The drawing under review shows one solid part. Ordinate dimensions are in mm from its lowest x, y, z. Coordinates: 2 decimals unless noted, no trailing zeros. Write each loop counter-clockwise with the first axis right and the second up, starting at its lowest first coordinate (ties: lowest second). Pieces come first, ordered by that corner, then holes. Notation, with made-up numbers: (67, 1.25) - (87, 1.25) arc R20 ccw to (87, 8.25) - close; hole circle Ø11 at (-17.75, -18). An arc over 180 degrees is marked (long way). Use a Markdown table: item, result.
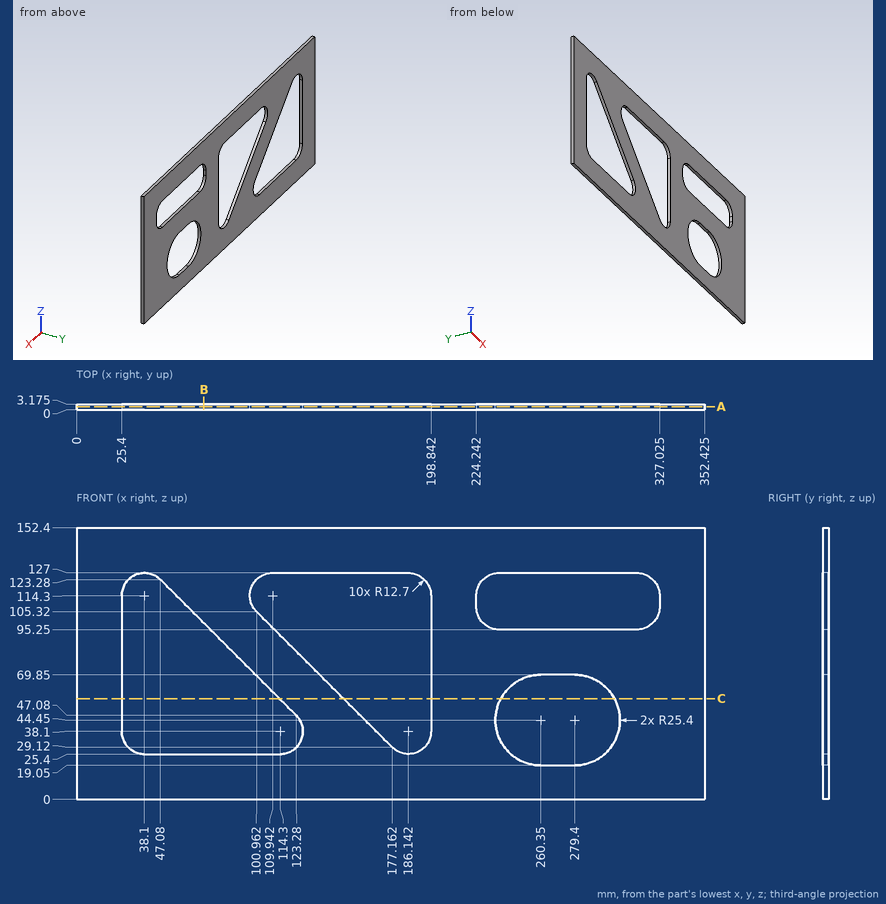
(1) Take a section at B-B on x = 71.5. Write out the cut boundary in (y, z) (1 decimal).
Determined:
| item | result |
|---|---|
| outline | (0, 0) - (3.2, 0) - (3.2, 25.4) - (0, 25.4) - close; (0, 98.9) - (3.2, 98.9) - (3.2, 152.4) - (0, 152.4) - close |
(2) For L1, parallel to X at y = 0.2, z = 97.5 (1 decimal); L2, parallel to X at y = 0.6, z = 29 (1 decimal); L3, parallel to X at y = 0.55, z = 73.5 (1 decimal), list the stretches that pass through material, from the lowest coordinate up. Write a range as from..to.
Determined:
| item | result |
|---|---|
| L1 | 0..25.4, 72.9..108.8, 198.8..229.7, 321.5..352.4 |
| L2 | 0..29.2, 123.2..177.3, 195..240.2, 299.6..352.4 |
| L3 | 0..25.4, 96.9..132.8, 198.8..352.4 |
(3) Take a section at C-C on z = 56.5. Write out the cut boundary in (x, y) (1 decimal), and give its area (3 significant figures).
Determined:
| item | result |
|---|---|
| outline | (0, 0) - (25.4, 0) - (25.4, 3.2) - (0, 3.2) - close; (113.9, 0) - (149.8, 0) - (149.8, 3.2) - (113.9, 3.2) - close; (198.8, 0) - (238, 0) - (238, 3.2) - (198.8, 3.2) - close; (301.8, 0) - (352.4, 0) - (352.4, 3.2) - (301.8, 3.2) - close |
| area | 480 mm2 |
(4) Take a section at A-A on y = 1.75. State how many separate pieces and enclosed holes the cut face has, and give its area (3 significant figures).
Determined:
| item | result |
|---|---|
| separate pieces | 1 |
| enclosed holes | 4 |
| area | 34,200 mm2 |
